Work out the finished part from the listing and answer in its coordinate system (mm). Coordinates: 2 decimals unless noted, no trailing zeros. Write each loop counter-clockwise with the first axis right and the second up, starting at its lowest first coordinate (ties: lowest second). Pieces come first, ordered by that corner, then holes. Notation, with made-up numbers: (-26, -23) - (-16, -23) arc R17 cw to (-16, 2) - close; hole circle Ø9 at (60, 32.25). An arc over 180 degrees is marked (long way). One line per item, written item: value.
```python
from build123d import *

# Parameters (mm, degrees)
BOSS_EXTRUDE1_DEPTH     = 1.5
CUT_EXTRUDE1_DEPTH      = 16
CUT_EXTRUDE1_DEPTH_BACK = 10.5
SKETCH2_R               = 3
SKETCH2_R_2             = 1.5


with BuildPart() as part:
    # Sketch1 → Boss-Extrude1 (new body)
    with BuildSketch(Plane(origin=(0, 0, 0), x_dir=(1, 0, 0), z_dir=(0, 1, 0))):
        with BuildLine():
            Line((0.449368076, 5.983148697), (40, 4.5))
            ThreePointArc((40, 4.5), (44.5, 0), (40, -4.5))
            Line((40, -4.5), (0.449368076, -5.983148697))
            ThreePointArc((0.449368076, -5.983148697), (-6, 0), (0.449368076, 5.983148697))
        make_face()
    extrude(amount=BOSS_EXTRUDE1_DEPTH)

    # Sketch2 → Cut-Extrude1 (cut, two sides: drawn at the far end of the back side and taken through both)
    with BuildSketch(Plane(origin=(0, 1.5, 0), x_dir=(1, 0, 0), z_dir=(0, 1, 0)).offset(-CUT_EXTRUDE1_DEPTH_BACK)):
        with Locations(Location((0, 0, 0), (0, 0, 270))):
            Circle(SKETCH2_R)
        with Locations(Location((40, 0, 0), (0, 0, 270))):
            Circle(SKETCH2_R_2)
    extrude(amount=CUT_EXTRUDE1_DEPTH + CUT_EXTRUDE1_DEPTH_BACK, mode=Mode.SUBTRACT)


solid = part.part
```
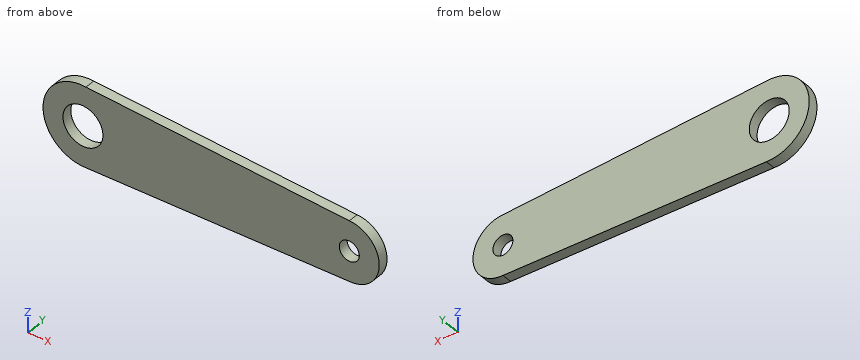
Item 1: Section B-B, the plane z = 0 is taken. Determine the outline of the cut face in (x, y).
Evaluation:
outline: (-6, 0) - (-3, 0) - (-3, 1.5) - (-6, 1.5) - close; (3, 0) - (38.5, 0) - (38.5, 1.5) - (3, 1.5) - close; (41.5, 0) - (44.5, 0) - (44.5, 1.5) - (41.5, 1.5) - close
Item 2: Section D-D, the plane z = -2 is taken. Determine the outline of the cut face in (x, y).
Evaluation:
outline: (-5.66, 0) - (-2.24, 0) - (-2.24, 1.5) - (-5.66, 1.5) - close; (2.24, 0) - (44.03, 0) - (44.03, 1.5) - (2.24, 1.5) - close
Item 3: Section A-A, the plane x = 0 is taken. Determine the outline of the cut face in (y, z), then the cut area to 3 significant figures.
Evaluation:
outline: (0, -6) - (1.5, -6) - (1.5, -3) - (0, -3) - close; (0, 3) - (1.5, 3) - (1.5, 6) - (0, 6) - close
area: 9.00 mm2
Item 4: Consider probe 1 along X at (y, z) = (0.45, 0); probe 2 along X at (y, z) = (1.25, -1.25); probe 3 along Z at (x, y) = (0, 0.6). Determine where each line is inside the solid, lowest interval first.
Evaluation:
probe 1: x = -6 to -3, 3 to 38.5, 41.5 to 44.5
probe 2: x = -5.87 to -2.73, 2.73 to 39.17, 40.83 to 44.32
probe 3: z = -6 to -3, 3 to 6
Item 5: Section C-C, the plane y = 1.2 is taken. Determine the outline of the cut face in (x, z), then the cut area to 3 significant figures.
Evaluation:
outline: (0.45, -5.98) - (40, -4.5) arc R4.5 ccw to (40, 4.5) - (0.45, 5.98) arc R6 ccw (long way) to start; hole circle Ø6 at (0, 0); hole circle Ø3 at (40, 0)
area: 473 mm2
